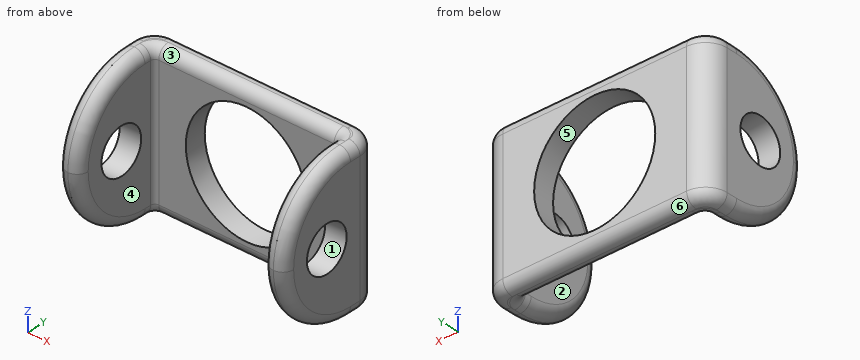
from build123d import *

# Parameters (mm, degrees)
SKETCH1_W           = 105
SKETCH1_H           = 70
SKETCH1_R           = 28
BOSS_EXTRUDE1_DEPTH = 10
SKETCH3_W           = 10
SKETCH3_H           = 70
BOSS_EXTRUDE2_DEPTH = 40
SKETCH5_R           = 10.5
CUT_EXTRUDE1_DEPTH  = 118.686022959
FILLET1_R           = 35
FILLET2_R           = 10
FILLET3_R           = 2
FILLET4_R           = 5


with BuildPart() as part:
    # Sketch1 → Boss-Extrude1 (new body)
    with BuildSketch(Plane(origin=(0, 0, 0), x_dir=(1, 0, 0), z_dir=(0, 1, 0))):
        Rectangle(SKETCH1_W, SKETCH1_H)
        with Locations(Location((0, 0, 0), (0, 0, 270))):
            Circle(SKETCH1_R, mode=Mode.SUBTRACT)
    extrude(amount=BOSS_EXTRUDE1_DEPTH)

    # Sketch3 → Boss-Extrude2 (add)
    with BuildSketch(Plane.XZ):
        with Locations((-47.5, 0)):
            Rectangle(SKETCH3_W, SKETCH3_H)
        with Locations((47.5, 0)):
            Rectangle(SKETCH3_W, SKETCH3_H)
    extrude(amount=BOSS_EXTRUDE2_DEPTH)

    # Sketch5 → Cut-Extrude1 (cut, through all)
    with BuildSketch(Plane(origin=(52.5, 0, 0), x_dir=(0, 0, -1), z_dir=(1, 0, 0))):
        with Locations((0, -17.5)):
            Circle(SKETCH5_R)
    extrude(amount=-CUT_EXTRUDE1_DEPTH, mode=Mode.SUBTRACT)

    # Fillet1
    fillet1_edges = [part.edges().sort_by_distance(p)[0] for p in [
        (47.5, -40, 35),
        (47.5, -40, -35),
        (-47.5, -40, 35),
        (-47.5, -40, -35),
    ]]
    fillet(fillet1_edges, radius=FILLET1_R - 0.0001)  # a hair under: the kernel refuses the full size

    # Fillet2
    fillet2_edges = [part.edges().sort_by_distance(p)[0] for p in [
        (52.5, 10, 0),
        (-52.5, 10, 0),
    ]]
    fillet(fillet2_edges, radius=FILLET2_R)

    # Fillet3
    fillet3_edges = [part.edges().sort_by_distance(p)[0] for p in [
        (-42.5, 0, 0),
        (42.5, 0, 0),
    ]]
    fillet(fillet3_edges, radius=FILLET3_R)

    # Fillet4
    fillet4_edges = [part.edges().sort_by_distance(p)[0] for p in [
        (-41.914213562, -0.585786438, 35),
        (-42.5, -29.748766631, 24.748766631),
        (-42.5, -29.748766631, -24.748766631),
        (-41.914213562, -0.585786438, -35),
        (0, 0, -35),
        (41.914213562, -0.585786438, -35),
        (42.5, -29.748766631, -24.748766631),
        (42.5, -29.748766631, 24.748766631),
        (41.914213562, -0.585786438, 35),
        (-49.571067812, 7.071067812, 35),
        (-52.5, -2.50005, 35),
        (-52.5, -29.748766631, 24.748766631),
        (-52.5, -29.748766631, -24.748766631),
        (-52.5, -2.50005, -35),
        (-49.571067812, 7.071067812, -35),
        (0, 10, -35),
        (49.571067812, 7.071067812, -35),
        (52.5, -2.50005, -35),
        (52.5, -29.748766631, -24.748766631),
        (52.5, -29.748766631, 24.748766631),
        (52.5, -2.50005, 35),
        (49.571067812, 7.071067812, 35),
        (0, 0, 35),
        (0, 10, 35),
        (-42.5, -3.50005, 35),
        (-42.5, -3.50005, -35),
        (42.5, -3.50005, -35),
        (42.5, -3.50005, 35),
    ]]
    fillet(fillet4_edges, radius=FILLET4_R - 0.0001)  # a hair under: the kernel refuses the full size


solid = part.part
Read the model definition and answer for the solid it produces. Units are mm, in the model's axes. Face numbers are marked on the shaded views. A direction names the side the tool comes from. Give positions to 0.01 mm unless a question says otherwise; leave off trailing zeros. Use a Markdown table: item, result.
Q1. Each of these flat-tipped pins is pushed along its axis until it touches: pin 1 (8 mm diameter, centred on x = 32.5, z = -10, fed in from -Y); pin 2 (1.5 mm diameter, centred on y = -32.5, z = -20.5, fed in from +X); pin 3 (1 mm diameter, centred on y = -32, z = 13.5, fed in from +X); pin 4 (1 mm diameter, centred on y = 4.5, z = 26, fed in from +X). Where does it stop, or does it pass through?
Solved:
| item | result |
|---|---|
| pin 1 | stops at y = 0 |
| pin 2 | stops at x = 51.02 |
| pin 3 | stops at x = 52.5 |
| pin 4 | stops at x = 51.67 |
Q2. Section B-B, the plane y = -13.5 is taken. Count the separate pieces of the cut face and the enclosed holes in it, then the cut area to 3 significant figures.
Solved:
| item | result |
|---|---|
| separate pieces | 4 |
| enclosed holes | 0 |
| area | 925 mm^2 |
Q3. Determine the mould class of the marked faces 4, 5 and 6 for opening direction Z: pulls with the +Z half, pulls with the -Z half, needs draft (parallel to the pull), parting line crosses it, or undercut.
Solved:
| item | result |
|---|---|
| face 4 | needs draft |
| face 5 | undercut |
| face 6 | pulls with the -Z half |
Q4. A tool of negligible diameter and unlimited length cuts with its end or side. For the marked faces 1, 2 and 3, from which of +Z, -Z, +X, -X, +Y, -Y can it reach the whole face along a straight path? Write none if from no direction.
Solved:
| item | result |
|---|---|
| face 1 | +X, -X |
| face 2 | +Z, -Z, -Y |
| face 3 | +Z, -Y |
Q5. Find the intervals of material crossed by line 1 along X through (y, z) = (-14, 28.5); line 2 along Y through (x, z) = (48.5, 0); line 3 along X through (y, z) = (-13.5, 32.5), in increasing order.
Solved:
| item | result |
|---|---|
| line 1 | x = -52.5 to -42.5, 42.5 to 52.5 |
| line 2 | y = -39.9 to -28, -7 to 8 |
| line 3 | x = -50.98 to -44.02, 44.02 to 50.98 |
